Here's how the part is built. I have some questions about the finished solid (model axes, mm). Round coordinates to 2 decimals unless told otherwise and drop trailing zeros. Order: outer loops, then holes, each group sorted by start corner. A loop starts at its lowest first (then second) coordinate and runs counter-clockwise, first axis right, second up.
Autodesk Inventor part; units mm, degrees
ref_plane "YZ Plane" through (0, 0, 0) normal (1, 0, 0) x (0, 1, 0)
ref_plane "XZ Plane" through (0, 0, 0) normal (0, 1, 0) x (-1, 0, 0)
ref_plane "XY Plane" through (0, 0, 0) normal (0, 0, 1) x (1, 0, 0)
sketch "Skizze1" plane through (0, 0, 0) normal (0, 0, 1) x (1, 0, 0)
  line L0 (-4.05, -4.05) -> (4.05, -4.05)
  line L1 (4.05, -4.05) -> (4.05, 4.05)
  line L2 (4.05, 4.05) -> (-4.05, 4.05)
  line L3 (-4.05, 4.05) -> (-4.05, -4.05)
  line L4 (-4.05, -4.05) -> (4.05, 4.05) construction
  line L5 (4.05, -4.05) -> (-4.05, 4.05) construction
  point P0 (0, 0)
  dimension "d0" = 8.1
extrude "Extrusion1" add sketch "Skizze1" along normal blind 7.5
sketch "Skizze3" plane through (0, 0, 7.5) normal (0, 0, 1) x (1, 0, 0)
  point P0 (0, 0)
  point P1 (0, 0)
hole "Bohrung1" at (0, 0, 7.5) direction (0, 0, -1) diameter 2 end through all
sketch "Skizze4" plane through (-4.05, 4.05, 0) normal (0, 1, 0) x (1, 0, 0)
  line L0 (8.1, 0) -> (0, 0) construction
  line L1 (0, 0) -> (0, -7.5) construction
  line L2 (8.1, -7.5) -> (0, -7.5) construction
  line L3 (8.1, 0) -> (8.1, -7.5) construction
  line L4 (8.1, -7.5) -> (0, -7.5)
  line L5 (4.05, -7.5) -> (4.05, 0) construction
  point P0 (4.05, -5.5)
  dimension "d11" = 2
hole "Bohrung2" at (0, 4.05, 5.5) direction (0, -1, 0) diameter 1.567 end through all
chamfer "Fase1" distance 1.5 angle 45 4 edges at (-4.05, 4.05, 3.75) (4.05, 4.05, 3.75) (-4.05, -4.05, 3.75) (4.05, -4.05, 3.75)
properties part number "Drehmomentuebertraeger_V4_1" material "Aluminium 6061"
1. If we mould it in two halves opening along Y, with no side actions, what happens to faces 1 (the flat face through (-3.3, 3.3, 3.7)), 2 (the flat face through (3.3, -3.3, 3.8)), 3 (the flat face through (-1, 1, 7.5)), 4 (the cylindrical face through (0, -1, 4))? For each: released by +Y, released by -Y, zero draft, split by the parting line, or undercut.
Evaluation:
face 1: released by +Y
face 2: released by -Y
face 3: zero draft
face 4: undercut
2. If we section it at B-B, the plane z = 3.75: Write out the boundary of the cut face in (x, y).
Evaluation:
outline: (-4.05, -2.55) - (-2.55, -4.05) - (2.55, -4.05) - (4.05, -2.55) - (4.05, 2.55) - (2.55, 4.05) - (-2.55, 4.05) - (-4.05, 2.55) - close; hole circle Ø2 at (0, 0)
3. If we section it at A-A, the plane y = 0: Write out the boundary of the cut face in (x, z).
Evaluation:
outline: (-4.05, 0) - (-1, 0) - (-1, 7.5) - (-4.05, 7.5) - close; (1, 0) - (4.05, 0) - (4.05, 7.5) - (1, 7.5) - close
4. I'm going to push a flat-ended pin straight in: P1, Ø1.8, axis at x = 0, y = 0, coming from the +Z side. Where does the tip first touch, or does it pass through?
Evaluation:
P1: passes through
5. If we section it at C-C, the plane x = 0: Write out the boundary of the cut face in (y, z).
Evaluation:
outline: (-4.05, 0) - (-1, 0) - (-1, 4.72) - (-4.05, 4.72) - close; (-4.05, 6.28) - (-1, 6.28) - (-1, 7.5) - (-4.05, 7.5) - close; (1, 0) - (4.05, 0) - (4.05, 4.72) - (1, 4.72) - close; (1, 6.28) - (4.05, 6.28) - (4.05, 7.5) - (1, 7.5) - close
6. I need wall thicknesses on probe 1 along X at (y, z) = (0, 5); probe 2 along Z at (x, y) = (0, -3); probe 3 along X at (y, z) = (-2.35, 5.5). Which ranges of each line are inside material? Lowest first, please.
Evaluation:
probe 1: x = -4.05 to -1, 1 to 4.05
probe 2: z = 0 to 4.72, 6.28 to 7.5
probe 3: x = -4.05 to -0.78, 0.78 to 4.05
7. If we section it at D-D, the plane z = 5.5: Write out the boundary of the cut face in (x, y), and give its area (4 significant figures).
Evaluation:
outline: (-4.05, -2.55) - (-2.55, -4.05) - (-0.78, -4.05) - (-0.78, -0.62) arc R1 cw to (-0.78, 0.62) - (-0.78, 4.05) - (-2.55, 4.05) - (-4.05, 2.55) - close; (0.78, -4.05) - (2.55, -4.05) - (4.05, -2.55) - (4.05, 2.55) - (2.55, 4.05) - (0.78, 4.05) - (0.78, 0.62) arc R1 cw to (0.78, -0.62) - close
area: 48.05 mm2
